Check sheet for the modelled part. Datum: model origin and axes. Units: mm. A direction names the side the tool comes from. Give positions to 0.01 mm unless a question says otherwise; leave off trailing zeros. Loops run counter-clockwise (first coordinate to the right, second up) from the corner with the lowest first, then second, coordinate; pieces in that order, holes last. Notation, with made-up numbers: M 53,-5 L 68,-5 A30 cw 68,20 Z; hole C 2.5,13.25 d2. An arc over 180 degrees is marked long. Put each result on its own line as item: value. Start each with the question number.
Autodesk Fusion 360 part; units mm, degrees
sketch "Sketch1" plane through (0, 0, 0) normal (0, 0, 1) x (1, 0, 0)
  line L0 (0, 0) -> (70, 0)
  line L1 (70, 0) -> (70, 60)
  line L2 (0, 60) -> (0, 0)
  line L3 (10, 15) -> (60, 15)
  line L4 (60, 15) -> (60, 30)
  line L5 (60, 30) -> (10, 30)
  line L6 (10, 30) -> (10, 15)
  circle A0 centre (35, 60) radius 20
  arc A1 (70, 60) -> (0, 60) centre (35, 60) ccw
  dimension "d1" = 70
  dimension "d2" = 60
  dimension "d5" = 15
  dimension "d6" = 50
  dimension "d10" = 10
  dimension "d11" = 15
  dimension "d15" = 40
  dimension "d16" = 35
extrude "Extrude1" add sketch "Sketch1" along normal blind 5
Q1. Depth check by flat-ended pin: P1, Ø2, axis at x = 54.5, z = 3.5, coming from the -Y side. Enter the tip coordinate at first touch or a pass-through.
Q2. Thickness scan on line 1 along Y through (x, z) = (35, 3.95); line 2 along X through (y, z) = (17.5, 4.4); line 3 along Y through (x, z) = (41.5, 0.7). Record the ranges inside material, lowest first. Write a range as [from, to].
Q3. Mould release check, pull along Y, two halves, no side actions. Record for faces 1 (the face through (35, 38, 5)), 2 (the face through (35, 15, 2)), 3 (the face through (34.23, 94.99, 2.46)): pulls with the +Y half, pulls with the -Y half, needs draft (parallel to the pull), parting line crosses it, or undercut.
Q4. Section check C-C, the plane z = 1.2. Record the cut outline in (x, y).
Q5. Section check D-D, the plane y = 48. Record the cut outline in (x, z).
Q6. Section check B-B, the plane x = 35. Record the cut outline in (y, z), then the cut area to 3 significant figures.
Q7. Section check A-A, the plane y = 27.5. Record the cut outline in (x, z), then the cut area to 3 significant figures.
Q8. Access from +Z, -Z, +X, -X, +Y, -Y to the whole of each face (thin tool, end or side, straight path). Record for faces 4 (the face through (70, 30, 2)), 5 (the face through (10, 23, 2)).
Found:
1. P1: stops at y = 0
2. line 1: y = [0, 15], [30, 40], [80, 95]
2. line 2: x = [0, 10], [60, 70]
2. line 3: y = [0, 15], [30, 41.09], [78.91, 94.39]
3. face 1: needs draft
3. face 2: undercut
3. face 3: pulls with the +Y half
4. outline: M 0,0 L 70,0 L 70,60 A35 ccw 0,60 Z; hole M 10,15 L 60,15 L 60,30 L 10,30 Z; hole C 35,60 d40
5. outline: M 0,0 L 19,0 L 19,5 L 0,5 Z; M 51,0 L 70,0 L 70,5 L 51,5 Z
6. outline: M 0,0 L 15,0 L 15,5 L 0,5 Z; M 30,0 L 40,0 L 40,5 L 30,5 Z; M 80,0 L 95,0 L 95,5 L 80,5 Z
6. area: 200 mm^2
7. outline: M 0,0 L 10,0 L 10,5 L 0,5 Z; M 60,0 L 70,0 L 70,5 L 60,5 Z
7. area: 100 mm^2
8. face 4: +Z, -Z, +X, +Y, -Y
8. face 5: +Z, -Z
